The listing builds one solid part. Answer for the finished solid, in the listing's coordinates (mm). Face numbers are marked on the shaded views. A direction names the side the tool comes from. Give positions to 0.01 mm unless a question says otherwise; leave off trailing zeros. Write each loop counter-clockwise with the first axis right and the second up, starting at its lowest first coordinate (ties: lowest second). Pieces come first, ordered by that corner, then holes.
```python
from build123d import *

# Parameters (mm, degrees)
SKETCH1_W               = 40
SKETCH1_H               = 29
BOSS_EXTRUDE1_DEPTH     = 20
FILLET2_R               = 6.5
SKETCH6_W               = 47.866272002
SKETCH6_H               = 35.823148672
CUT_EXTRUDE6_DEPTH      = 7.5
SHELL1_T                = -2
SKETCH7_R               = 2.95
CUT_EXTRUDE7_DEPTH      = 1
CUT_EXTRUDE7_DEPTH_BACK = 41
SKETCH8_R               = 2.95
CUT_EXTRUDE8_DEPTH      = 30
CUT_EXTRUDE10_DEPTH     = 3.3


with BuildPart() as part:
    # Sketch1 → Boss-Extrude1 (new body)
    with BuildSketch(Plane(origin=(0, 0, 0), x_dir=(1, 0, 0), z_dir=(0, 1, 0))):
        Rectangle(SKETCH1_W, SKETCH1_H)
    extrude(amount=BOSS_EXTRUDE1_DEPTH)

    # Fillet2
    fillet2_edges = [part.edges().sort_by_distance(p)[0] for p in [
        (-20, 20, 0),
        (0, 20, 14.5),
        (20, 20, 0),
        (0, 0, 14.5),
        (-20, 0, 0),
        (0, 0, -14.5),
        (20, 0, 0),
        (20, 10, 14.5),
        (-20, 10, 14.5),
        (-20, 10, -14.5),
        (20, 10, -14.5),
        (0, 20, -14.5),
    ]]
    fillet(fillet2_edges, radius=FILLET2_R)

    # Sketch6 → Cut-Extrude6 (cut, through all)
    with BuildSketch(Plane(origin=(0, 13.5, 0), x_dir=(1, 0, 0), z_dir=(0, 1, 0))):
        Rectangle(SKETCH6_W, SKETCH6_H)
    extrude(amount=CUT_EXTRUDE6_DEPTH, mode=Mode.SUBTRACT)

    # Shell1
    shell1_openings = [part.faces().sort_by_distance(p)[0] for p in [
        (0, 13.5, 0),
    ]]
    offset(amount=SHELL1_T, openings=shell1_openings, kind=Kind.INTERSECTION)

    # Sketch7 → Cut-Extrude7 (cut, two sides)
    with BuildSketch(Plane(origin=(20, 0, 0), x_dir=(0, 0, -1), z_dir=(1, 0, 0))) as cut_extrude7_sk:
        with Locations((4, 10)):
            Circle(SKETCH7_R)
        with Locations((-4, 10)):
            Circle(SKETCH7_R)
    extrude(amount=CUT_EXTRUDE7_DEPTH, mode=Mode.SUBTRACT)
    extrude(cut_extrude7_sk.sketch, amount=-CUT_EXTRUDE7_DEPTH_BACK, mode=Mode.SUBTRACT)

    # Sketch8 → Cut-Extrude8 (cut, through all)
    with BuildSketch(Plane.XY.offset(14.5)):
        with Locations((-6.75, 10)):
            Circle(SKETCH8_R)
        with Locations(Location((6.75, 10, 0), (0, 0, 180))):  # turned: the seam where the file's is
            Circle(SKETCH8_R)
    extrude(amount=-CUT_EXTRUDE8_DEPTH, mode=Mode.SUBTRACT)

    # Sketch10 → Cut-Extrude10 (cut)
    with BuildSketch(Plane(origin=(0, 13.5, 0), x_dir=(1, 0, 0), z_dir=(0, 1, 0))):
        with BuildLine():
            ThreePointArc((-18.5, -8), (-17.035533906, -11.535533906), (-13.5, -13))
            ThreePointArc((-13.5, -13), (-13, -13.5), (-13.5, -14))
            ThreePointArc((-13.5, -14), (-17.742640687, -12.242640687), (-19.5, -8))
            ThreePointArc((-19.5, -8), (-19, -7.5), (-18.5, -8))
        make_face()
        with BuildLine():
            ThreePointArc((-13.5, 13), (-17.035533906, 11.535533906), (-18.5, 8))
            ThreePointArc((-18.5, 8), (-19, 7.5), (-19.5, 8))
            ThreePointArc((-19.5, 8), (-17.742640687, 12.242640687), (-13.5, 14))
            ThreePointArc((-13.5, 14), (-13, 13.5), (-13.5, 13))
        make_face()
        with BuildLine():
            ThreePointArc((18.5, 8), (17.035533906, 11.535533906), (13.5, 13))
            ThreePointArc((13.5, 13), (13, 13.5), (13.5, 14))
            ThreePointArc((13.5, 14), (17.742640687, 12.242640687), (19.5, 8))
            ThreePointArc((19.5, 8), (19, 7.5), (18.5, 8))
        make_face()
        with BuildLine():
            ThreePointArc((13.5, -13), (17.035533906, -11.535533906), (18.5, -8))
            ThreePointArc((18.5, -8), (19, -7.5), (19.5, -8))
            ThreePointArc((19.5, -8), (17.742640687, -12.242640687), (13.5, -14))
            ThreePointArc((13.5, -14), (13, -13.5), (13.5, -13))
        make_face()
    extrude(amount=-CUT_EXTRUDE10_DEPTH, mode=Mode.SUBTRACT)


solid = part.part
```
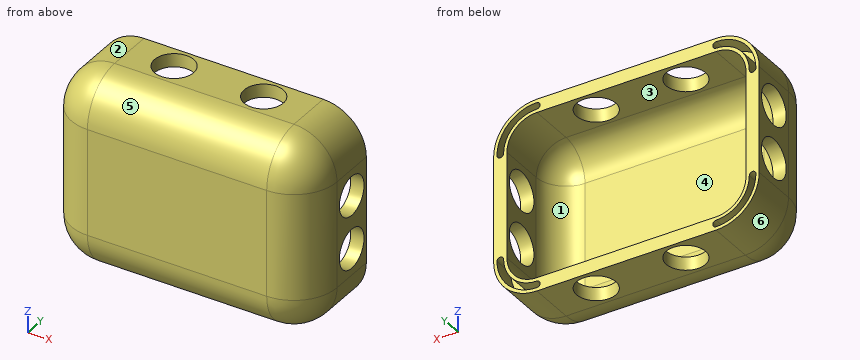
Item 1: Which of the six approach directions +Z, -Z, +X, -X, +Y, -Y give full straight-line access (tool end or side, diameter ignored) to the marked faces 1 and 2?
Conclusion:
face 1: +Y
face 2: +Z, -X, +Y, -Y
Item 2: A cutting plane is placed at D-D, the plane x = -1.5. Give the vertices of the cut face in (y, z), plus the area to 3 significant figures.
Conclusion:
outline: (0, -8) arc R6.5 ccw to (6.5, -14.5) - (13.5, -14.5) - (13.5, -12.5) - (6.5, -12.5) arc R4.5 cw to (2, -8) - (2, 8) arc R4.5 cw to (6.5, 12.5) - (13.5, 12.5) - (13.5, 14.5) - (6.5, 14.5) arc R6.5 ccw to (0, 8) - close
area: 94.6 mm2
Item 3: A cutting plane is placed at A-A, the plane z = 4. Give the vertices of the cut face in (x, y), plus the area to 3 significant figures.
Conclusion:
outline: (-20, 6.5) arc R6.5 ccw to (-13.5, 0) - (13.5, 0) arc R6.5 ccw to (20, 6.5) - (20, 7.05) - (18, 7.05) - (18, 6.5) arc R4.5 cw to (13.5, 2) - (-13.5, 2) arc R4.5 cw to (-18, 6.5) - (-18, 7.05) - (-20, 7.05) - close; (-20, 12.95) - (-18, 12.95) - (-18, 13.5) - (-20, 13.5) - close; (18, 12.95) - (20, 12.95) - (20, 13.5) - (18, 13.5) - close
area: 93.0 mm2
Item 4: Determine the mould class of the marked faces 3, 4, 5 and 6 for opening direction X: pulls with the +X half, pulls with the -X half, needs draft (parallel to the pull), parting line crosses it, or undercut.
Conclusion:
face 3: undercut
face 4: undercut
face 5: needs draft
face 6: pulls with the -X half
Item 5: A cutting plane is placed at B-B, the plane x = 6.75. Give the vertices of the cut face in (y, z).
Conclusion:
outline: (0, -8) arc R6.5 ccw to (6.5, -14.5) - (7.05, -14.5) - (7.05, -12.5) - (6.5, -12.5) arc R4.5 cw to (2, -8) - (2, 8) arc R4.5 cw to (6.5, 12.5) - (7.05, 12.5) - (7.05, 14.5) - (6.5, 14.5) arc R6.5 ccw to (0, 8) - close; (12.95, -14.5) - (13.5, -14.5) - (13.5, -12.5) - (12.95, -12.5) - close; (12.95, 12.5) - (13.5, 12.5) - (13.5, 14.5) - (12.95, 14.5) - close
Item 6: Each of these flat-tipped pins is pushed along its axis until it touches: P1, Ø2, axis at y = 8.5, z = -3, coming from the +X side; P2, Ø8, axis at x = 2.5, z = -3, coming from the +Y side; P3, Ø7, axis at y = 10, z = 4, coming from the -X side; P4, Ø6, axis at x = 7.5, z = -6.5, coming from the +Y side. Where does it stop, or does it pass through?
Conclusion:
P1: passes through
P2: stops at y = 2
P3: stops at x = -20
P4: stops at y = 2.26
Item 7: Consider probe 1 along Z at (x, y) = (13.5, 7.5); probe 2 along X at (y, z) = (11.5, 9); probe 3 along X at (y, z) = (12.75, -7.75). Determine where each line is inside the solid, lowest interval first.
Conclusion:
probe 1: z = -14.5 to -12.5, 12.5 to 14.5
probe 2: x = -19.92 to -19.42, -18.4 to -17.89, 17.89 to 18.4, 19.42 to 19.92
probe 3: x = -20 to -19.43, -18.57 to -18, 18 to 18.57, 19.43 to 20
Item 8: A cutting plane is placed at C-C, the plane y = 4. Give the vertices of the cut face in (x, z).
Conclusion:
outline: (-19.5, -8) arc R6 ccw to (-13.5, -14) - (13.5, -14) arc R6 ccw to (19.5, -8) - (19.5, 8) arc R6 ccw to (13.5, 14) - (-13.5, 14) arc R6 ccw to (-19.5, 8) - close; hole (-17.24, -8) arc R3.74 ccw to (-13.5, -11.74) - (13.5, -11.74) arc R3.74 ccw to (17.24, -8) - (17.24, 8) arc R3.74 ccw to (13.5, 11.74) - (-13.5, 11.74) arc R3.74 ccw to (-17.24, 8) - close
